Verification items for the finished model (mm, model axes). A direction names the side the tool comes from. Round coordinates to 2 decimals unless told otherwise and drop trailing zeros. Write each loop counter-clockwise with the first axis right and the second up, starting at its lowest first coordinate (ties: lowest second). Pieces come first, ordered by that corner, then holes. Notation, with made-up numbers: (77, 28) - (131, 28) arc R20 cw to (131, 48) - close; hole circle Ø1 at (9, 86.25). An arc over 180 degrees is marked (long way). Answer as a JSON object with one key per item and string values. Group by question number.
1) Section check A-A (x = 52.5). Enter the section's corners in (y, z), then the cut area to 3 significant figures.
2) Section check C-C (y = 23). Enter the section's corners in (x, z), then the cut area to 3 significant figures.
3) Go/stop test with a flat-tipped pin: pin 1 Ø6 at (x, z) = (54.5, 4) entering from +Y. Record where the tip stops, or that it passes through.
4) Thickness scan on line 1 (X direction, y = 9, z = 4.75); line 2 (Y direction, x = 59, z = 2.75); line 3 (Z direction, x = 48, y = 3.5). Record the ranges inside material, lowest first.
5) Mould release check, pull along Z, two halves, no side actions. Record for faces 1 (the conical face through (5.566, 40.759, 5.981)), 2 (the flat face through (47, 29, 12)), 3 (the flat face through (33, 0, 6)): +Z half, -Z half, draft (parallel to the pull), parting line (faces both ways), or undercut.
6) Section check B-B (y = 13). Enter the section's corners in (x, z), then the cut area to 3 significant figures.
7) Set-up check for faces 4 (the cylindrical face through (41.69, 49.4, 6.96)), 5 (the flat face through (50, 47, 6)), 6 (the cylindrical face through (50.31, 7.6, 6.96)), 7 (the flat face through (53, 25.5, 6)): record each of +Z, -Z, +X, -X, +Y, -Y from which the full face is reachable in a straight line by a thin tool's end or side.
8) Section check D-D (x = 25). Enter the section's corners in (y, z).
```python
from build123d import *

# Parameters (mm, degrees)
ESBO_O1_R                                   = 21
RESSALTO_EXTRUS_O1_DEPTH                    = 12
ESBO_O2_W                                   = 20
ESBO_O2_H                                   = 1
CORTE_EXTRUS_O1_DEPTH                       = 88.281154896
BROCA_DE_ROSQUEAR_PARA_TARRAXA_DE_M81_D     = 6.8
BROCA_DE_ROSQUEAR_PARA_TARRAXA_DE_M81_DEPTH = 25
BROCA_DE_ROSQUEAR_PARA_TARRAXA_DE_M81_TIP   = 2.042926105
BROCA_DE_ROSQUEAR_PARA_TARRAXA_DE_M62_D     = 5
BROCA_DE_ROSQUEAR_PARA_TARRAXA_DE_M62_DEPTH = 15
BROCA_DE_ROSQUEAR_PARA_TARRAXA_DE_M62_TIP   = 1.502151548
BROCA_DE_ROSQUEAR_PARA_TARRAXA_DE_M63_D     = 5
BROCA_DE_ROSQUEAR_PARA_TARRAXA_DE_M63_DEPTH = 15
BROCA_DE_ROSQUEAR_PARA_TARRAXA_DE_M63_TIP   = 1.502151548


with BuildPart() as part:
    # Esboço1 → Ressalto-extrusão1 (new body)
    with BuildSketch(Plane.XY):
        Polygon((0, 0), (0, 57), (50, 57), (50, 37), (65, 37), (65, 0), align=None)
        with Locations((25, 25)):
            Circle(ESBO_O1_R, mode=Mode.SUBTRACT)
    extrude(amount=RESSALTO_EXTRUS_O1_DEPTH)

    # Esboço2 → Corte-extrusão1 (cut, through all)
    with BuildSketch(Plane.XY.offset(12)):
        with Locations((55, 25)):
            Rectangle(ESBO_O2_W, ESBO_O2_H)
    extrude(amount=-CORTE_EXTRUS_O1_DEPTH, mode=Mode.SUBTRACT)

    # Broca de rosquear para tarraxa de M81
    with Locations(Plane(origin=(0, 37, 0), x_dir=(1, 0, 0), z_dir=(0, 1, 0))):
        with Locations((57.5, -6)):
            Hole(BROCA_DE_ROSQUEAR_PARA_TARRAXA_DE_M81_D / 2, depth=BROCA_DE_ROSQUEAR_PARA_TARRAXA_DE_M81_DEPTH)
            with Locations((0, 0, -(BROCA_DE_ROSQUEAR_PARA_TARRAXA_DE_M81_DEPTH + BROCA_DE_ROSQUEAR_PARA_TARRAXA_DE_M81_TIP / 2))):  # 118° drill point
                Cone(0, BROCA_DE_ROSQUEAR_PARA_TARRAXA_DE_M81_D / 2, BROCA_DE_ROSQUEAR_PARA_TARRAXA_DE_M81_TIP, mode=Mode.SUBTRACT)

    # Broca de rosquear para tarraxa de M62
    with Locations(Plane(origin=(0, 57, 0), x_dir=(1, 0, 0), z_dir=(0, 1, 0))):
        with Locations((6, -6), (44, -6)):
            Hole(BROCA_DE_ROSQUEAR_PARA_TARRAXA_DE_M62_D / 2, depth=BROCA_DE_ROSQUEAR_PARA_TARRAXA_DE_M62_DEPTH)
            with Locations((0, 0, -(BROCA_DE_ROSQUEAR_PARA_TARRAXA_DE_M62_DEPTH + BROCA_DE_ROSQUEAR_PARA_TARRAXA_DE_M62_TIP / 2))):  # 118° drill point
                Cone(0, BROCA_DE_ROSQUEAR_PARA_TARRAXA_DE_M62_D / 2, BROCA_DE_ROSQUEAR_PARA_TARRAXA_DE_M62_TIP, mode=Mode.SUBTRACT)

    # Broca de rosquear para tarraxa de M63
    with Locations(Plane(origin=(0, 0, 0), x_dir=(-1, 0, 0), z_dir=(0, -1, 0))):
        with Locations((-4, -6), (-48, -6)):
            Hole(BROCA_DE_ROSQUEAR_PARA_TARRAXA_DE_M63_D / 2, depth=BROCA_DE_ROSQUEAR_PARA_TARRAXA_DE_M63_DEPTH)
            with Locations((0, 0, -(BROCA_DE_ROSQUEAR_PARA_TARRAXA_DE_M63_DEPTH + BROCA_DE_ROSQUEAR_PARA_TARRAXA_DE_M63_TIP / 2))):  # 118° drill point
                Cone(0, BROCA_DE_ROSQUEAR_PARA_TARRAXA_DE_M63_D / 2, BROCA_DE_ROSQUEAR_PARA_TARRAXA_DE_M63_TIP, mode=Mode.SUBTRACT)


solid = part.part
```
Returned:
{
 "1": {"outline": "(0, 0) - (24.5, 0) - (24.5, 12) - (0, 12) - close; (25.5, 0) - (37, 0) - (37, 12) - (25.5, 12) - close", "area": "432 mm2"},
 "2": {"outline": "(0, 0) - (4.1, 0) - (4.1, 12) - (0, 12) - close; (45.9, 0) - (65, 0) - (65, 12) - (45.9, 12) - close; hole circle Ø6.8 at (57.5, 6)", "area": "242 mm2"},
 "3": {"pin 1": "y = 37"},
 "4": {"line 1": "0 to 1.83, 6.17 to 11.4, 38.6 to 45.83, 50.17 to 65", "line 2": "0 to 24.5, 25.5 to 37", "line 3": "0 to 3.5, 8.5 to 12"},
 "5": {"face 1": "undercut", "face 2": "+Z half", "face 3": "draft"},
 "6": {"outline": "(0, 0) - (7.77, 0) - (7.77, 12) - (0, 12) - close; (42.23, 0) - (65, 0) - (65, 12) - (42.23, 12) - close; hole circle Ø5 at (4, 6); hole circle Ø5 at (48, 6); hole circle Ø6.8 at (57.5, 6)", "area": "291 mm2"},
 "7": {"face 4": "+Y", "face 5": "+Z, -Z, +X, +Y", "face 6": "-Y", "face 7": "+Z, -Z, +X"},
 "8": {"outline": "(0, 0) - (4, 0) - (4, 12) - (0, 12) - close; (46, 0) - (57, 0) - (57, 12) - (46, 12) - close"}
}
